```python
from build123d import *

# Parameters (mm, degrees)
SKETCH1_W           = 50
SKETCH1_H           = 25
BOSS_EXTRUDE2_DEPTH = 15
FILLET1_R           = 4
FILLET2_R           = 4
SHELL1_T            = -1.2
SKETCH2_R           = 8.25
CUT_EXTRUDE1_DEPTH  = 58.579857589
SKETCH3_R           = 1.5
BOSS_EXTRUDE3_DEPTH = 7
SKETCH6_R           = 0.5
CUT_EXTRUDE3_DEPTH  = 3
CUT_EXTRUDE6_DEPTH  = 1
SKETCH9_R           = 4
CUT_EXTRUDE15_DEPTH = 1.2
SKETCH13_R          = 2.5
CUT_EXTRUDE16_DEPTH = 58.579857676


with BuildPart() as part:
    # Sketch1 → Boss-Extrude2 (new body)
    with BuildSketch(Plane(origin=(0, 0, 0), x_dir=(1, 0, 0), z_dir=(0, 1, 0))):
        with Locations((25, 12.5)):
            Rectangle(SKETCH1_W, SKETCH1_H)
    extrude(amount=BOSS_EXTRUDE2_DEPTH)

    # Fillet1
    fillet1_edges = [part.edges().sort_by_distance(p)[0] for p in [
        (0, 7.5, -25),
        (50, 7.5, -25),
        (50, 7.5, 0),
        (0, 7.5, 0),
    ]]
    fillet(fillet1_edges, radius=FILLET1_R)

    # Fillet2
    fillet2_edges = [part.edges().sort_by_distance(p)[0] for p in [
        (50, 15, -12.5),
        (25, 15, 0),
        (0, 15, -12.5),
        (25, 15, -25),
        (48.828427125, 15, -23.828427125),
        (1.171572875, 15, -23.828427125),
        (1.171572875, 15, -1.171572875),
        (48.828427125, 15, -1.171572875),
    ]]
    fillet(fillet2_edges, radius=FILLET2_R)

    # Shell1
    shell1_openings = [part.faces().sort_by_distance(p)[0] for p in [
        (25, 0, -12.5),
    ]]
    offset(amount=SHELL1_T, openings=shell1_openings, kind=Kind.INTERSECTION)

    # Sketch2 → Cut-Extrude1 (cut, through all)
    with BuildSketch(Plane.XZ.offset(-13.8)):
        with Locations(Location((38, -12.5, 0), (0, 0, 345.858889766))):
            Circle(SKETCH2_R)
        with Locations(Location((12, -12.5, 0), (0, 0, 194.141110234))):
            Circle(SKETCH2_R)
    extrude(amount=-CUT_EXTRUDE1_DEPTH, mode=Mode.SUBTRACT)

    # Sketch3 → Boss-Extrude3 (add)
    with BuildSketch(Plane.XZ.offset(-13.8)):
        with Locations(Location((46.25, -21.25, 0), (0, 0, 99.594068224))):
            Circle(SKETCH3_R)
        with Locations(Location((3.75, -21.25, 0), (0, 0, 80.405931773))):
            Circle(SKETCH3_R)
        with Locations(Location((3.75, -3.75, 0), (0, 0, 80.405943008))):
            Circle(SKETCH3_R)
        with Locations(Location((46.25, -3.75, 0), (0, 0, 99.594068235))):
            Circle(SKETCH3_R)
    extrude(amount=BOSS_EXTRUDE3_DEPTH)

    # Sketch6 → Cut-Extrude3 (cut)
    with BuildSketch(Plane.XZ.offset(-6.8)):
        with Locations(Location((46.25, -3.75, 0), (0, 0, 270))):
            Circle(SKETCH6_R)
        with Locations(Location((46.25, -21.25, 0), (0, 0, 270))):
            Circle(SKETCH6_R)
        with Locations(Location((3.75, -21.25, 0), (0, 0, 270))):
            Circle(SKETCH6_R)
        with Locations(Location((3.75, -3.75, 0), (0, 0, 270))):
            Circle(SKETCH6_R)
    extrude(amount=-CUT_EXTRUDE3_DEPTH, mode=Mode.SUBTRACT)

    # Sketch8 → Cut-Extrude6 (cut)
    with BuildSketch(Plane.XZ):
        with BuildLine():
            Line((0.6, -4), (0.6, -21))
            ThreePointArc((0.6, -21), (1.595836944, -23.404163056), (4, -24.4))
            Line((4, -24.4), (46, -24.4))
            ThreePointArc((46, -24.4), (48.404163056, -23.404163056), (49.4, -21))
            Line((49.4, -21), (49.4, -4))
            ThreePointArc((49.4, -4), (48.404163056, -1.595836944), (46, -0.6))
            Line((46, -0.6), (4, -0.6))
            ThreePointArc((4, -0.6), (1.595836944, -1.595836944), (0.6, -4))
        make_face()
    extrude(amount=-CUT_EXTRUDE6_DEPTH, mode=Mode.SUBTRACT)

    # Sketch9 → Cut-Extrude15 (cut)
    with BuildSketch(Plane(origin=(0, 0, -25), x_dir=(-1, 0, 0), z_dir=(0, 0, -1))):
        with Locations((-25, 6)):
            Circle(SKETCH9_R)
    extrude(amount=-CUT_EXTRUDE15_DEPTH, mode=Mode.SUBTRACT)

    # Sketch13 → Cut-Extrude16 (cut, through all)
    with BuildSketch(Plane.XZ.offset(-13.8)):
        with Locations(Location((25, -12.5, 0), (0, 0, 270))):
            Circle(SKETCH13_R)
    extrude(amount=-CUT_EXTRUDE16_DEPTH, mode=Mode.SUBTRACT)


solid = part.part
```
CAD build for the part. Positions are in the model's coordinates, mm. A direction names the side the tool comes from. Give positions to 0.01 mm unless a question says otherwise; leave off trailing zeros. Write each loop counter-clockwise with the first axis right and the second up, starting at its lowest first coordinate (ties: lowest second). Pieces come first, ordered by that corner, then holes. Notation, with made-up numbers: M 89,-11.75 L 135,-11.75 A20 ccw 135,15.25 Z; hole C 78,4.25 d4. An arc over 180 degrees is marked long. Return JSON: item names as keys, results as strings. Group by question number.
(1) Drill centre lines: L1, parallel to X at y = 8.35, z = -3.75; L2, parallel to Z at x = 44, y = 7.25; L3, parallel to Z at x = 46.25, y = 8.85. Where is each one in solid material? Low to high. Write a range as [from, to].
(2) Band-saw the part on C-C (x = 25). Give the cut face in (y, z).
(3) Band-saw the part on B-B (y = 1.5). Give the cut face in (x, z).
(4) Band-saw the part on D-D (y = 12.5). Give the cut face in (x, z).
(5) 3-axis set-ups, long thin cutter, end or side, ignore diameter. For faces 4 (the face through (24.7, 1.8, -25)), 5 (the face through (3, 6.8, -4)): which of +Z, -Z, +X, -X, +Y, -Y reach the whole face in a straight line?
(6) Mould opens along X. For faces 1 (the face through (1.141, 5.577, -23.797)), 2 (the face through (24.9, 0, -24.6)), 3 (the face through (44.816, 10.349, -4.19)) say: pulls with the +X half, pulls with the -X half, needs draft (parallel to the pull), parting line crosses it, or undercut.
(7) Flat gauge pins, fed straight in: pin 1 Ø3.5 at (x, z) = (4, -21.5) entering from -Y; pin 2 Ø6 at (x, z) = (25, -12.5) entering from -Y; pin 3 Ø1 at (x, y) = (45, 12.5) entering from -Z. Where does each tip first touch, or does it go through?
(8) Band-saw the part on A-A (x = 12). Give the cut face in (y, z), and give its area (3 significant figures).
Entries:
{
 "1": {"L1": "x = [0.01, 1.21], [2.25, 3.25], [4.25, 5.25], [44.75, 45.75], [46.75, 47.75], [48.79, 49.99]", "L2": "z = [-25, -23.8], [-1.2, 0]", "L3": "z = [-24.99, -23.79], [-22.75, -21.75], [-20.75, -19.75], [-5.25, -4.25], [-3.25, -2.25], [-1.21, -0.01]"},
 "2": {"outline": "M 0,-25 L 2,-25 L 2,-23.8 L 1,-23.8 L 1,-24.4 L 0,-24.4 Z; M 0,-0.6 L 1,-0.6 L 1,-1.2 L 11,-1.2 A2.8 cw 13.8,-4 L 13.8,-10 L 15,-10 L 15,-4 A4 ccw 11,0 L 0,0 Z; M 10,-25 L 11,-25 A4 ccw 15,-21 L 15,-15 L 13.8,-15 L 13.8,-21 A2.8 cw 11,-23.8 L 10,-23.8 Z"},
 "3": {"outline": "M 0,-21 A4 ccw 4,-25 L 46,-25 A4 ccw 50,-21 L 50,-4 A4 ccw 46,0 L 4,0 A4 ccw 0,-4 Z; hole M 1.2,-21 A2.8 ccw 4,-23.8 L 46,-23.8 A2.8 ccw 48.8,-21 L 48.8,-4 A2.8 ccw 46,-1.2 L 4,-1.2 A2.8 ccw 1.2,-4 Z"},
 "4": {"outline": "M 0.29,-21 A3.71 ccw 4,-24.71 L 46,-24.71 A3.71 ccw 49.71,-21 L 49.71,-4 A3.71 ccw 46,-0.29 L 4,-0.29 A3.71 ccw 0.29,-4 Z; C 3.75,-21.25 d3; C 3.75,-3.75 d3; C 46.25,-21.25 d3; C 46.25,-3.75 d3; hole M 1.64,-21 A2.36 ccw 4,-23.36 L 46,-23.36 A2.36 ccw 48.36,-21 L 48.36,-4 A2.36 ccw 46,-1.64 L 4,-1.64 A2.36 ccw 1.64,-4 Z"},
 "5": {"face 4": "-Z, +X, -X, +Y, -Y", "face 5": "-Y"},
 "6": {"face 1": "pulls with the -X half", "face 2": "needs draft", "face 3": "undercut"},
 "7": {"pin 1": "stops at y = 6.8", "pin 2": "stops at y = 13.8", "pin 3": "stops at z = -24.87"},
 "8": {"outline": "M 0,-25 L 11,-25 A4 ccw 15,-21 L 15,-20.75 L 13.8,-20.75 L 13.8,-21 A2.8 cw 11,-23.8 L 1,-23.8 L 1,-24.4 L 0,-24.4 Z; M 0,-0.6 L 1,-0.6 L 1,-1.2 L 11,-1.2 A2.8 cw 13.8,-4 L 13.8,-4.25 L 15,-4.25 L 15,-4 A4 ccw 11,0 L 0,0 Z", "area": "38.6 mm^2"}
}
